Read the model definition and answer for the solid it produces. Units are mm, in the model's axes. Face numbers are marked on the shaded views. A direction names the side the tool comes from. Give positions to 0.01 mm unless a question says otherwise; leave off trailing zeros. Order: outer loops, then holes, each group sorted by start corner. A loop starts at its lowest first (then second) coordinate and runs counter-clockwise, first axis right, second up. Notation, with made-up numbers: (9.25, -37) - (19.25, -37) arc R23 ccw to (19.25, -27) - close; hole circle Ø11 at (83.25, 6). An arc over 180 degrees is marked (long way). Write each question's results on one line, items separated by ' | '. Start each with the question number.
Q1. Find the intervals of material crossed by line 1 along Y through (x, z) = (17, 9); line 2 along X through (y, z) = (33, 1); line 3 along Z through (x, y) = (15.5, 53.5), in increasing order. Write a range as from..to.
Q2. A tool of negligible diameter and unlimited length cuts with its end or side. For the marked faces 1, 2 and 3, from which of +Z, -Z, +X, -X, +Y, -Y can it reach the whole face along a straight path? Write none if from no direction.
Q3. For a pull along X with two mould halves and no side action, classify the marked faces 4, 5, 6 and 7 as +X half, -X half, draft (parallel to the pull), parting line (faces both ways), or undercut.
Q4. Find section A-A on z = 17.75. Give the vertices of the cut face in (x, y), and give its area (3 significant figures).
Q5. Flat-ended cylindrical pins translate along their axes: P1, Ø12, axis at x = 24, z = 13, coming from the -Y side; P2, Ø16.5, axis at x = 20, y = 21.5, coming from the +Z side; P3, Ø1.5, axis at y = 27, z = 3.5, coming from the +X side; P4, Ø2.5, axis at y = 37.5, z = 3.5, coming from the -X side. Find the tip coordinate at first contact, or state that the pin passes through.
Q6. Find section D-D on x = 13.5. Give the vertices of the cut face in (y, z), and give its area (3 significant figures).
Q7. Find section B-B on x = 18.5. Give the vertices of the cut face in (y, z), and give its area (3 significant figures).
Q8. Find section C-C on z = 4.25. Give the vertices of the cut face in (x, y).
from build123d import *

# Parameters (mm, degrees)
PAD_DEPTH     = 5
SKETCH001_W   = 37
SKETCH001_H   = 5
SKETCH001_W_2 = 15
PAD001_DEPTH  = 20


with BuildPart() as part:
    # Sketch → Pad (new body)
    with BuildSketch(Plane.XY):
        Polygon((0, 5), (0, 0), (37, 0), (37, 5), (26, 5), (26, 65), (11, 65), (11, 5), align=None)
        Polygon((16, 5), (21, 5), (21, 55), (16.000076, 55), align=None, mode=Mode.SUBTRACT)
    extrude(amount=PAD_DEPTH)

    # Sketch001 → Pad001 (join)
    with BuildSketch(Plane.XY):
        with Locations((18.5, 2.5)):
            Rectangle(SKETCH001_W, SKETCH001_H)
        with Locations((18.5, 62.5)):
            Rectangle(SKETCH001_W_2, SKETCH001_H)
    extrude(amount=PAD001_DEPTH)


solid = part.part
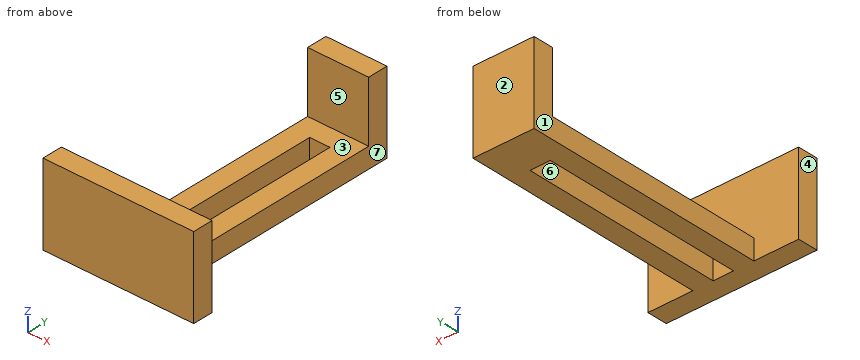
Working result:
1) line 1: 0..5, 60..65 | line 2: 11..16, 21..26 | line 3: 0..5
2) face 1: +Z, -Z, -X, +Y | face 2: +Z, -Z, +X, -X, +Y | face 3: +Z, +X, -X
3) face 4: -X half | face 5: draft | face 6: undercut | face 7: +X half
4) outline: (0, 0) - (37, 0) - (37, 5) - (0, 5) - close; (11, 60) - (26, 60) - (26, 65) - (11, 65) - close | area: 260 mm²
5) P1: y = 0 | P2: z = 5 | P3: x = 26 | P4: x = 11
6) outline: (0, 0) - (65, 0) - (65, 20) - (60, 20) - (60, 5) - (5, 5) - (5, 20) - (0, 20) - close | area: 475 mm²
7) outline: (0, 0) - (5, 0) - (5, 20) - (0, 20) - close; (55, 0) - (65, 0) - (65, 20) - (60, 20) - (60, 5) - (55, 5) - close | area: 225 mm²
8) outline: (0, 0) - (37, 0) - (37, 5) - (26, 5) - (26, 65) - (11, 65) - (11, 5) - (0, 5) - close; hole (16, 5) - (21, 5) - (21, 55) - (16, 55) - close
